Autodesk Inventor part; units mm, degrees
ref_plane "YZ Plane" through (0, 0, 0) normal (1, 0, 0) x (0, 1, 0)
ref_plane "XZ Plane" through (0, 0, 0) normal (0, 1, 0) x (-1, 0, 0)
ref_plane "XY Plane" through (0, 0, 0) normal (0, 0, 1) x (1, 0, 0)
sketch "Szkic1" plane through (0, 0, 0) normal (1, 0, 0) x (0, 1, 0)
  line L0 (-32.5, 103) -> (32.5, 103)
  line L1 (38.5, 97) -> (38.5, -97)
  line L2 (32.5, -103) -> (-32.5, -103)
  line L3 (-38.5, -97) -> (-38.5, 97)
  line L4 (-38.5, 103) -> (38.5, -103) construction
  arc A0 (32.5, -103) -> (38.5, -97) centre (32.5, -97) ccw
  arc A1 (-32.5, 103) -> (-38.5, 97) centre (-32.5, 97) ccw
  arc A2 (-38.5, -97) -> (-32.5, -103) centre (-32.5, -97) ccw
  arc A3 (38.5, 97) -> (32.5, 103) centre (32.5, 97) ccw
  point P0 (0, 0)
  dimension "d3" = 6
extrude "Płyta1" add sketch "Szkic1" along normal blind 3
sketch "Szkic2" plane through (3, 0, 0) normal (1, 0, 0) x (0, 0, -1)
  line L0 (-97, 38.5) -> (97, 38.5)
  line L1 (-103, -32.5) -> (-103, 32.5)
  line L2 (103, 32.5) -> (103, -32.5)
  line L3 (97, -38.5) -> (-97, -38.5)
  point P0 (0, 0)
  point P1 (-53, 25.5)
  point P2 (53, 25.5)
  point P3 (53, -25.5)
  point P4 (-53, -25.5)
  dimension "d5" = 13
  dimension "d6" = 50
  dimension "d7" = 50
  dimension "d8" = 13
  dimension "d9" = 50
  dimension "d10" = 13
  dimension "d11" = 13
  dimension "d12" = 50
hole "Otwór1" at (3, -25.5, 53) at (3, 25.5, 53) at (3, 25.5, -53) at (3, -25.5, -53) direction (-1, 0, 0) diameter 5.5 depth 3 tip angle 118
sketch "Sketch3" plane through (3, 0, 0) normal (1, 0, 0) x (0, 0, -1)
  line L0 (103, 32.5) -> (103, -32.5)
  line L1 (97, -38.5) -> (-97, -38.5)
  point P0 (0, 0)
  point P1 (45, 9.5)
  dimension "d20" = 58
  dimension "d40" = 48
hole "Hole2" at (3, 9.5, -45) direction (-1, 0, 0) diameter 12 depth 3 tip angle 118
sketch "Sketch4" plane through (3, 0, 0) normal (1, 0, 0) x (0, 0, -1)
  circle A0 centre (45, 9.5) radius 6
  point P0 (0, 0)
  point P1 (33, 9.5)
  dimension "d28" = 12
  dimension "d29" = 0
hole "Hole3" at (3, 9.5, -33) direction (-1, 0, 0) diameter 4.3 depth 3 tip angle 118
pattern_circular "Circular Pattern1" count 4 over 360 about axis through (1.5, 9.5, -45) along (1, 0, 0) of "Hole3"
equation "\"d18\" = Grubość"
equation "\"d26\" = Grubość"
equation "\"d35\" = Grubość"
equation "\"d4\" = Grubość"
equation "\"PromieńGięcia\" = Grubość"
equation "\"SzerokośćGięciaPodcięcia\" = Grubość"
equation "\"GłębokośćGięciaPodcięcia\" = 0.5 * Grubość"
equation "\"RozmiarPodcięciaNarożnika\" = 4 * Grubość"
equation "\"MinimalnaPozostałość\" = 2 * Grubość"
equation "\"PromieńPrzejścia\" = PromieńGięcia"
equation "\"Rozmiar_promienia_Jacobiego\" = PromieńGięcia"
equation "\"Wielk_odstępu\" = Grubość"
properties part number "ZaslepkaObudowa2"
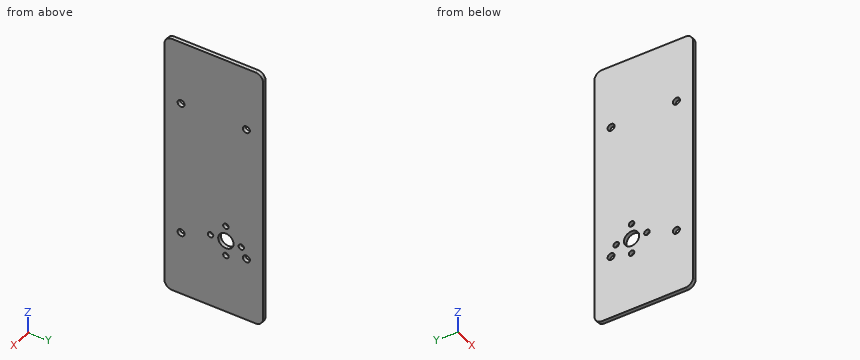
Here's how the part is built. I have some questions about the finished solid (model axes, mm). Coordinates: 2 decimals unless noted, no trailing zeros. Order: outer loops, then holes, each group sorted by start corner. A loop starts at its lowest first (then second) coordinate and runs counter-clockwise, first axis right, second up. Notation, with made-up numbers: (-31, 33) - (-21, 33) arc R35 ccw to (-21, 67) - close; hole circle Ø3 at (83.5, 33). An arc over 180 degrees is marked (long way). One line per question, with ' | ' between items. Start each with the question number.
1. If we section it at A-A (z = 53): Write out the boundary of the cut face in (x, y), and give its area (3 significant figures).
2. If we section it at D-D (x = 1.75): Give the number of separate pieces and of enclosed holes in the cut face, and give its area (3 significant figures).
3. If we section it at B-B (y = 9.5): Write out the boundary of the cut face in (x, z), and give its area (3 significant figures).
4. If we section it at C-C (y = -25.5): Write out the boundary of the cut face in (x, z).
5. Please list where these lines run through material, in increasing order: line 1 along Z through (x, y) = (0.85, 25.5); line 2 along Y through (x, z) = (1.35, 53); line 3 along Y through (x, z) = (2, -57). Write a range as [from, to].
Model answer:
1) outline: (0, -38.5) - (3, -38.5) - (3, -28.25) - (0, -28.25) - close; (0, -22.75) - (3, -22.75) - (3, 22.75) - (0, 22.75) - close; (0, 28.25) - (3, 28.25) - (3, 38.5) - (0, 38.5) - close | area: 198 mm²
2) separate pieces: 1 | enclosed holes: 9 | area: 15,600 mm²
3) outline: (0, -103) - (3, -103) - (3, -59.15) - (0, -59.15) - close; (0, -54.85) - (3, -54.85) - (3, -51) - (0, -51) - close; (0, -39) - (3, -39) - (3, -35.15) - (0, -35.15) - close; (0, -30.85) - (3, -30.85) - (3, 103) - (0, 103) - close | area: 556 mm²
4) outline: (0, -103) - (3, -103) - (3, -55.75) - (0, -55.75) - close; (0, -50.25) - (3, -50.25) - (3, 50.25) - (0, 50.25) - close; (0, 55.75) - (3, 55.75) - (3, 103) - (0, 103) - close
5) line 1: z = [-103, -55.75], [-50.25, 50.25], [55.75, 103] | line 2: y = [-38.5, -28.25], [-22.75, 22.75], [28.25, 38.5] | line 3: y = [-38.5, 7.35], [11.65, 38.5]
